```python
from build123d import *

# Parameters (mm, degrees)
F0_W     = 38.1
F0_H     = 31.75
F1_DEPTH = 25.4
F2_W     = 12.7
F2_H     = 6.35
F3_DEPTH = 25.401
F4_W     = 38.1
F4_H     = 8.8702891953
F5_DEPTH = 6.35


# Not quite as in the source:
# - a length typed as a fraction of an inch, garbled in the dataset ("3 / 203.2 mm" for 3/8 in), is restored


with BuildPart() as f1:
    # F0 (on Front) → F1 (new body)
    with BuildSketch(Plane.XZ):
        with Locations((19.05, 15.875)):
            Rectangle(F0_W, F0_H)
    extrude(amount=F1_DEPTH)

    # F2 (on face) → F3 (cut, through all)
    with BuildSketch(Plane.XZ.offset(25.4)):
        with Locations((19.5667292759, 3.175)):
            Rectangle(F2_W, F2_H)
    extrude(amount=-F3_DEPTH, mode=Mode.SUBTRACT)

    # F4 (on face) → F5 (cut)
    with BuildSketch(Plane.XY.offset(31.75)):
        with Locations((19.05, -11.620078003)):
            Rectangle(F4_W, F4_H)
    extrude(amount=-F5_DEPTH, mode=Mode.SUBTRACT)


solid = f1.part
```
The model under review builds one solid part; all positions refer to its coordinate system, in mm. A direction names the side the tool comes from. Give positions to 0.01 mm unless a question says otherwise; leave off trailing zeros. Write each loop counter-clockwise with the first axis right and the second up, starting at its lowest first coordinate (ties: lowest second). Pieces come first, ordered by that corner, then holes. Notation, with made-up numbers: (-27, -4.75) -> (0, -4.75) arc R21 ccw to (0, 16.25) -> close; hole circle Ø11 at (-14.5, 50). An arc over 180 degrees is marked (long way). Put each result on its own line as item: value.
(1) The part is to be moulded in two halves that separate along Y. For faces 4 (the flat face through (19, -7.185, 29)), 5 (the flat face through (19, -25.4, 16)), 6 (the flat face through (13.217, -13, 3)), say which applies: pulls with the +Y half, pulls with the -Y half, needs draft (parallel to the pull), parting line crosses it, or undercut.
Results are:
face 4: undercut
face 5: pulls with the -Y half
face 6: needs draft
(2) Tool access review of faces 1 (the flat face through (19, -12, 25.4)), 2 (the flat face through (19, -13, 6.35)), 3 (the flat face through (7, -13, 0)): name each direction out of +Z, -Z, +X, -X, +Y, -Y from which nothing blocks a thin tool from reaching the whole face with its end or side.
Results are:
face 1: +Z, +X, -X
face 2: -Z, +Y, -Y
face 3: -Z, +X, -X, +Y, -Y
(3) We need section A-A, the plane z = 5. Give the boundary of the cut face in (x, y).
Results are:
outline: (0, -25.4) -> (13.22, -25.4) -> (13.22, 0) -> (0, 0) -> close; (25.92, -25.4) -> (38.1, -25.4) -> (38.1, 0) -> (25.92, 0) -> close
(4) To check wall thickness, follow probe 1 along Y at (x, z) = (23.5, 29); probe 2 along X at (y, z) = (-24, 6); probe 3 along Z at (x, y) = (24, -19). State the ranges of each line that lie inside material, in increasing order. Write a range as from..to.
Results are:
probe 1: -25.4..-16.06, -7.18..0
probe 2: 0..13.22, 25.92..38.1
probe 3: 6.35..31.75
(5) We need section D-D, the plane z = 26.5. Give the boundary of the cut face in (x, y), and give its area (3 significant figures).
Results are:
outline: (0, -25.4) -> (38.1, -25.4) -> (38.1, -16.06) -> (0, -16.06) -> close; (0, -7.18) -> (38.1, -7.18) -> (38.1, 0) -> (0, 0) -> close
area: 630 mm²
(6) We need section C-C, the plane x = 5.5. Give the boundary of the cut face in (y, z).
Results are:
outline: (-25.4, 0) -> (0, 0) -> (0, 31.75) -> (-7.18, 31.75) -> (-7.18, 25.4) -> (-16.06, 25.4) -> (-16.06, 31.75) -> (-25.4, 31.75) -> close
(7) For pin 1 Ø8 at (x, y) = (7.5, -11.5) entering from -Z; pin 2 Ø2.5 at (x, y) = (21.5, -12) entering from +Z, all flat-tipped, find the tip position at first contact; note any pin that passes through.
Results are:
pin 1: z = 0
pin 2: z = 25.4
(8) We need section B-B, the plane y = -8.25. Give the boundary of the cut face in (x, z).
Results are:
outline: (0, 0) -> (13.22, 0) -> (13.22, 6.35) -> (25.92, 6.35) -> (25.92, 0) -> (38.1, 0) -> (38.1, 25.4) -> (0, 25.4) -> close
